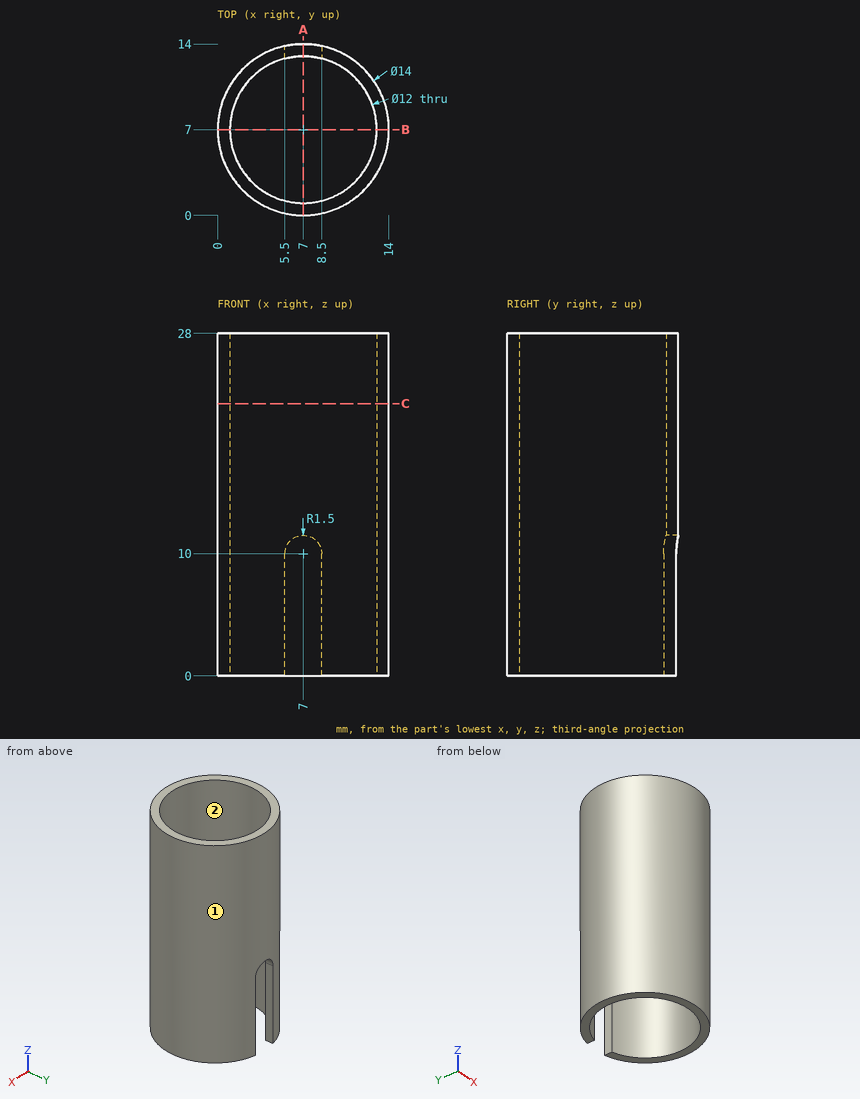
The figure shows three views and two pictorial views of one solid part (mm, origin at its lowest corner). Answer the questions. Round coordinates to 2 decimals unless told otherwise and drop trailing zeros. Order: outer loops, then holes, each group sorted by start corner. A loop starts at its lowest first (then second) coordinate and runs counter-clockwise, first axis right, second up.
Q1. Given pin 1 Ø0.8 at (y, z) = (13.5, 6) entering from -X; pin 2 Ø1 at (x, z) = (8.5, 8.5) entering from +Y; pin 3 Ø2 at (y, z) = (8.5, 16.5) entering from +X, each flat-ended and moving along its own axis, determine where each tip first touches the part or whether it passes through.
Solution:
pin 1: stops at x = 3.57
pin 2: stops at y = 13.84
pin 3: stops at x = 13.98
Q2. The mould has two halves that part along X. Classify the marked faces 1 and 2: pulls with the +X half, pulls with the -X half, needs draft (parallel to the pull), parting line crosses it, or undercut.
Solution:
face 1: parting line crosses it
face 2: undercut
Q3. A cutting plane is placed at A-A, the plane x = 7. Determine the outline of the cut face in (y, z), then the cut area to 3 significant figures.
Solution:
outline: (0, 0) - (1, 0) - (1, 28) - (0, 28) - close; (13, 11.5) - (14, 11.5) - (14, 28) - (13, 28) - close
area: 44.5 mm2
Q4. Find the intervals of material crossed by line 1 along Y through (x, z) = (7, 15.75); line 2 along Y through (x, z) = (12.5, 23.5); line 3 along X through (y, z) = (3.5, 26.75), in increasing order.
Solution:
line 1: y = 0 to 1, 13 to 14
line 2: y = 2.67 to 4.6, 9.4 to 11.33
line 3: x = 0.94 to 2.13, 11.87 to 13.06
Q5. A cutting plane is placed at C-C, the plane z = 22.25. Determine the outline of the cut face in (x, y), then the cut area to 3 significant figures.
Solution:
outline: circle Ø14 at (7, 7); hole circle Ø12 at (7, 7)
area: 40.8 mm2
Q6. A cutting plane is placed at B-B, the plane y = 7. Determine the outline of the cut face in (x, z), then the cut area to 3 significant figures.
Solution:
outline: (0, 0) - (1, 0) - (1, 28) - (0, 28) - close; (13, 0) - (14, 0) - (14, 28) - (13, 28) - close
area: 56.0 mm2
